```python
from build123d import *

# Parameters (mm, degrees)
SKETCH_1_W          = 40
SKETCH_1_H          = 85
EXTRUDE_1_DEPTH     = 5
SKETCH_2_W          = 25
SKETCH_2_H          = 85
EXTRUDE_2_DEPTH     = 2.5
EXTRUDE_START       = -7.5
SKETCH_5_W          = 38
SKETCH_5_H          = 85
EXTRUDE_3_DEPTH     = 7.5
SKETCH_3_R          = 3.4
CUT_EXTRUDE_1_DEPTH = 95.074438611
SKETCH_6_R          = 3.4
CUT_EXTRUDE_2_DEPTH = 95.074438611
FILLET_1_R          = 2
FILLET_2_R          = 2
SKETCH_7_W          = 63
SKETCH_7_H          = 17.986542749
CUT_EXTRUDE_3_DEPTH = 44
FILLET_3_R          = 2
EXTRUDE_4_DEPTH     = 39
FILLET_4_R          = 2


with BuildPart() as part:
    # 草图1 → 凸台-拉伸1 (new body)
    with BuildSketch(Plane(origin=(0, 0, 0), x_dir=(1, 0, 0), z_dir=(0, 1, 0))):
        with Locations((20, -42.5)):
            Rectangle(SKETCH_1_W, SKETCH_1_H)
    extrude(amount=EXTRUDE_1_DEPTH)

    # 草图2 → 凸台-拉伸2 (add)
    with BuildSketch(Plane(origin=(0, 5, 0), x_dir=(1, 0, 0), z_dir=(0, 1, 0))):
        with Locations((12.5, -42.5)):
            Rectangle(SKETCH_2_W, SKETCH_2_H)
    extrude(amount=EXTRUDE_2_DEPTH)

    # 草图5 → 凸台-拉伸3 (add)
    with BuildSketch(Plane.XZ.offset(EXTRUDE_START)):
        with Locations((-19, 42.5)):
            Rectangle(SKETCH_5_W, SKETCH_5_H)
    extrude(amount=EXTRUDE_3_DEPTH)

    # 草图3 → 切除-拉伸1 (cut, through all)
    with BuildSketch(Plane(origin=(0, 5, 0), x_dir=(1, 0, 0), z_dir=(0, 1, 0))):
        with Locations(Location((32.361090949, -75, 0), (0, 0, 270))):
            Circle(SKETCH_3_R)
    extrude(amount=-CUT_EXTRUDE_1_DEPTH, mode=Mode.SUBTRACT)

    # 草图6 → 切除-拉伸2 (cut, through all)
    with BuildSketch(Plane(origin=(0, 5, 0), x_dir=(1, 0, 0), z_dir=(0, 1, 0))):
        with Locations(Location((32.361090949, -10, 0), (0, 0, 270))):
            Circle(SKETCH_6_R)
    extrude(amount=-CUT_EXTRUDE_2_DEPTH, mode=Mode.SUBTRACT)

    # 圆角1
    fillet_1_edges = [part.edges().sort_by_distance(p)[0] for p in [
        (-6.5, 7.5, 85),
        (-38, 7.5, 42.5),
    ]]
    fillet(fillet_1_edges, radius=FILLET_1_R)

    # 圆角2
    # the kernel refuses this fillet: 2 mm, written as the material it takes off along each edge
    with BuildSketch(Plane(origin=(-36, 5.5, 83), x_dir=(0, 0, 1), z_dir=(-1, 0, 0))) as fillet_2_piece_1_section:
        Polygon((0, 0), (FILLET_2_R, 0), (FILLET_2_R, FILLET_2_R), (0, FILLET_2_R), align=None)
    fillet_2_piece_1 = extrude(amount=FILLET_2_R, mode=Mode.PRIVATE)
    fillet_2_piece_1 = fillet_2_piece_1 - Plane(origin=(-36, 5.5, 83), x_dir=(0, -0.7071067811865475, -0.7071067811865475), z_dir=(-1, 0, 0)) * Sphere(FILLET_2_R, mode=Mode.PRIVATE)
    add(fillet_2_piece_1, mode=Mode.SUBTRACT)
    with BuildSketch(Plane(origin=(-36, 7.5, 0), x_dir=(0, -1, 0), z_dir=(1, 0, 0))) as fillet_2_piece_2:
        with BuildLine():
            CenterArc((FILLET_2_R, -FILLET_2_R), FILLET_2_R, 90, 90)
            Line((0, -FILLET_2_R), (0, 0))
            Line((0, 0), (FILLET_2_R, 0))
        make_face()
    extrude(amount=66, mode=Mode.SUBTRACT)
    with BuildSketch(Plane(origin=(-38, 5.5, 85), x_dir=(0, 0, -1), z_dir=(0, -1, 0)), Plane(origin=(-38, 5.5, 0), x_dir=(1, 0, 0), z_dir=(0, -1, 0))) as fillet_2_piece_3:
        with BuildLine():
            CenterArc((FILLET_2_R, FILLET_2_R), FILLET_2_R, 180, 90)
            Line((0, FILLET_2_R), (0, 0))
            Line((0, 0), (FILLET_2_R, 0))
        make_face()
    extrude(amount=10.5, mode=Mode.SUBTRACT)
    with BuildSketch(Plane(origin=(-36, 5.5, 0), x_dir=(-1, 0, 0), z_dir=(0, -1, 0))) as fillet_2_piece_4:
        with BuildLine():
            CenterArc((2 - FILLET_2_R, -FILLET_2_R), FILLET_2_R, 0, 90)
            Line((2, -FILLET_2_R), (2, 0))
            Line((2, 0), (2 - FILLET_2_R, 0))
        make_face()
    revolve(axis=Axis((-36, 5.5, 0), (0, 0, -1)), revolution_arc=90, mode=Mode.SUBTRACT)

    # 草图7 → 切除-拉伸3 (cut)
    with BuildSketch(Plane.XY.offset(85)):
        with Locations((-6.5, 8.993271375)):
            Rectangle(SKETCH_7_W, SKETCH_7_H)
    extrude(amount=-CUT_EXTRUDE_3_DEPTH, mode=Mode.SUBTRACT)

    # 圆角3
    fillet_3_edges = [part.edges().sort_by_distance(p)[0] for p in [
        (-37.414213562, 6.914213562, 41),
        (-5.5, 7.5, 41),
        (-38, 2.75, 41),
    ]]
    fillet(fillet_3_edges, radius=FILLET_3_R)

    # 草图8 → 凸台-拉伸4 (add)
    with BuildSketch(Plane.ZY.offset(38)):
        Polygon((-1.392069631, 5), (2, 5), (2, 5.5), (2, 7.5), (-2.284139263, 7.5), (-2.284139263, 39), (-4.784139263, 39), (-4.784139263, 7.572997811), (-4.784139263, 5), align=None)
    extrude(amount=-EXTRUDE_4_DEPTH)

    # 圆角4
    fillet_4_edges = [part.edges().sort_by_distance(p)[0] for p in [
        (-38, 23.25, -2.284139263),
        (-38, 7.5, -0.142069631),
    ]]
    fillet(fillet_4_edges, radius=FILLET_4_R)


solid = part.part
```
Geometry check sheet. Reference: the model listing, model coordinates, mm. A direction names the side the tool comes from. Round coordinates to 2 decimals unless told otherwise and drop trailing zeros. Loops run counter-clockwise (first coordinate to the right, second up) from the corner with the lowest first, then second, coordinate; pieces in that order, holes last. Notation, with made-up numbers: (84.25, 83.25) - (103.25, 83.25) arc R28 ccw to (103.25, 107.25) - close; hole circle Ø10 at (-9, -6). An arc over 180 degrees is marked (long way). Use a Markdown table: item, result.
Q1. Go/stop test with flat-tipped pins: P1, Ø4, axis at y = 2.5, z = 66.5, coming from the -X side; P2, Ø4.5, axis at x = 7, y = 3.5, coming from the +Z side; P3, Ø9.5, axis at x = -11, y = 18.5, coming from the +Z side; P4, Ø3.5, axis at y = 19.5, z = -0.5, coming from the +X side. Record where each tip stops, or that it passes through.
Solutions:
| item | result |
|---|---|
| P1 | stops at x = 25 |
| P2 | stops at z = 41 |
| P3 | stops at z = -2.28 |
| P4 | passes through |
Q2. Cross-section at A-A on z = 75. Record the cut outline in (x, y).
Solutions:
| item | result |
|---|---|
| outline | (25, 0) - (28.96, 0) - (28.96, 5) - (25, 5) - close; (35.76, 0) - (40, 0) - (40, 5) - (35.76, 5) - close |
Q3. Access from +Z, -Z, +X, -X, +Y, -Y to the whole of each face (thin tool, end or side, straight path). Record for faces 1 (the flat face through (25, 2, 63)), 2 (the cylindrical face through (12.83, 6.9, 0.57)), 3 (the cylindrical face through (-37.43, 2.54, 0.6)), 4 (the cylindrical face through (-37.43, 6.9, 20.76)), 5 (the flat face through (25, 6, 21)).
Solutions:
| item | result |
|---|---|
| face 1 | +Z, -X, +Y, -Y |
| face 2 | -Z, +X, +Y |
| face 3 | -Z, -X, -Y |
| face 4 | +Z, -X, +Y |
| face 5 | +Z, -Z, +X, +Y |
Q4. Cross-section at C-C on z = 32. Record the cut outline in (x, y).
Solutions:
| item | result |
|---|---|
| outline | (-38, 0) - (40, 0) - (40, 5) - (25, 5) - (25, 7.5) - (-36, 7.5) arc R2 ccw to (-38, 5.5) - close |
Q5. Cross-section at B-B on x = -15. Record the cut outline in (y, z), plus the area to 3 significant figures.
Solutions:
| item | result |
|---|---|
| outline | (0, 0) - (5, 0) - (5, -4.78) - (39, -4.78) - (39, -2.28) - (7.5, -2.28) - (7.5, 39) arc R2 ccw to (5.5, 41) - (0, 41) - close |
| area | 397 mm2 |
Q6. Material ranges on line 1 (X direction, y = 3.6, z = 75); line 2 (Z direction, x = 30, y = 2.5); line 3 (Y direction, x = 6, z = 8.5), recorded low to high.
Solutions:
| item | result |
|---|---|
| line 1 | x = 25 to 28.96, 35.76 to 40 |
| line 2 | z = 0 to 7.55, 12.45 to 72.55, 77.45 to 85 |
| line 3 | y = 0 to 7.5 |
Q7. Cross-section at D-D on y = 13.5. Record the cut outline in (x, z), plus the area to 3 significant figures.
Solutions:
| item | result |
|---|---|
| outline | (-38, -4.78) - (1, -4.78) - (1, -2.28) - (-36, -2.28) arc R2 ccw to (-38, -4.28) - close |
| area | 96.6 mm2 |
